```python
from build123d import *

# Parameters (mm, degrees)
EXTRUDE_1_DEPTH = 131.5


with BuildPart() as part:
    # 草图1 → 凸台-拉伸1 (new, symmetric)
    with BuildSketch(Plane(origin=(0, 0, 0), x_dir=(1, 0, 0), z_dir=(0, 1, 0))):
        with BuildLine():
            Line((-76.837904128, -58.81687225), (-76.837904128, 125.19937152))
            Line((-76.837904128, 125.19937152), (144.166689092, 149.345372478))
            Line((144.166689092, 149.345372478), (144.166689092, -36.597164955))
            add(Edge.make_bspline(
                [(-76.837904128, -58.81687225), (-9.541749974, 14.78234011), (93.359068004, -119.986931913), (144.166689092, -36.597164955)],
                knots=[0, 0, 0, 0, 1, 1, 1, 1], degree=3))
        make_face()
    extrude(amount=EXTRUDE_1_DEPTH, both=True)


solid = part.part
```
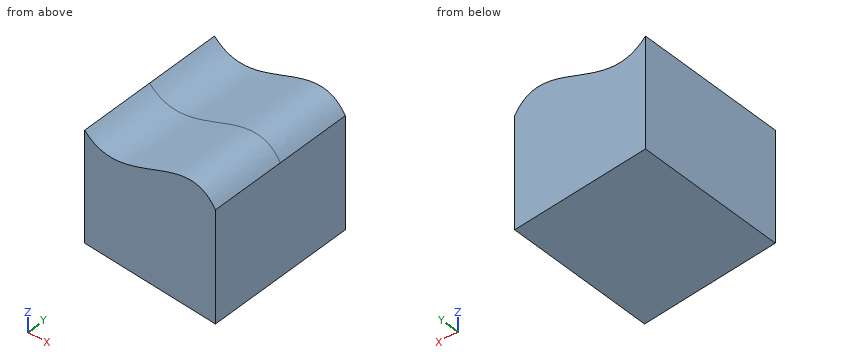
Read the model definition and answer for the solid it produces. Units are mm, in the model's axes. Coordinates: 2 decimals unless noted, no trailing zeros. Loops run counter-clockwise (first coordinate to the right, second up) from the corner with the lowest first, then second, coordinate; pieces in that order, holes last. Notation, with made-up numbers: (-38.75, -37.75) -> (-34.75, -37.75) arc R20 cw to (-34.75, -15.75) -> close; hole circle Ø3 at (-25.75, 35). An arc over 180 degrees is marked (long way). Return JSON: item names as keys, results as strings.
Item 1: Find section A-A (z = -132.5). Determine the outline of the cut face in (x, y), plus the area to 3 significant figures.
Answers:
{"outline": "(-10.02, -131.5) -> (144.17, -131.5) -> (144.17, 131.5) -> (-10.02, 131.5) -> close", "area": "40,600 mm2"}
Item 2: Flat-ended cylindrical pins translate along their axes: P1, Ø1.5, axis at x = 59, y = 20.5, coming from the -Z side; P2, Ø1, axis at x = 1, y = 32, coming from the -Z side. Find the tip coordinate at first contact, or state that the pin passes through.
Answers:
{"P1": "stops at z = -140.12", "P2": "stops at z = -133.76"}
Item 3: Find the intervals of material crossed by probe 1 along Z at (x, y) = (18, -61); probe 2 along Z at (x, y) = (20, -34.5), in increasing order.
Answers:
{"probe 1": "z = -135.56 to 44.02", "probe 2": "z = -135.78 to 44.65"}
